from build123d import *


with BuildPart() as part:
    # Sketch1 → Revolve1 (revolve)
    with BuildSketch(Plane.XY):
        with BuildLine():
            Line((10.15, 9.35), (10.15, 11.15))
            ThreePointArc((10.15, 11.15), (9.608147545, 12.458147545), (8.3, 13))
            Line((8.3, 13), (8.3, 14))
            Line((8.3, 14), (0, 14))
            Line((0, 14), (0, 13))
            ThreePointArc((0, 13), (-1.308147545, 12.458147545), (-1.85, 11.15))
            Line((-1.85, 11.15), (-1.85, 9.35))
            ThreePointArc((-1.85, 9.35), (-1.308147545, 8.041852455), (0, 7.5))
            Line((0, 7.5), (0, 6.5))
            Line((0, 6.5), (8.3, 6.5))
            Line((8.3, 6.5), (8.3, 7.5))
            ThreePointArc((8.3, 7.5), (9.608147545, 8.041852455), (10.15, 9.35))
        make_face()
    revolve(axis=Axis((-8.833016473, 0, 0), (1, 0, 0)))


solid = part.part
Verification items for the finished model (mm, model axes). A direction names the side the tool comes from. Coordinates: 2 decimals unless noted, no trailing zeros. Order: outer loops, then holes, each group sorted by start corner. A loop starts at its lowest first (then second) coordinate and runs counter-clockwise, first axis right, second up. Notation, with made-up numbers: M 79.25,65.5 L 122.25,65.5 A24 cw 122.25,93.5 Z; hole C 2.5,26.25 d10. An arc over 180 degrees is marked long. One line per item, written item: value. Start each with the question number.
Item 1: Sectioned sample at C-C on x = 7.5. Record the cut outline in (y, z), then the cut area to 3 significant figures.
Item 2: Thickness scan on probe 1 along Z at (x, y) = (3.75, 0); probe 2 along X at (y, z) = (-3.5, -8.5); probe 3 along Y at (x, z) = (5.25, 3). Record the ranges inside material, lowest first.
Item 3: Access from +Z, -Z, +X, -X, +Y, -Y to the whole of each face (thin tool, end or side, straight path). Record for faces 1 (the cylindrical face through (4.208, -5.158, -3.955)), 2 (the flat face through (8.3, -9.3, -9.3)).
Item 4: Mould release check, pull along Z, two halves, no side actions. Record for faces 3 (the flat face through (0, -6, 3)), 4 (the cylindrical face through (4.092, 12.932, -5.362)), 5 (the flat face through (0, 9.3, -9.3)): pulls with the +Z half, pulls with the -Z half, needs draft (parallel to the pull), parting line crosses it, or undercut.
Item 5: Depth check by flat-ended pin: P1, Ø2, axis at x = 2, z = 8, coming from the +Y side; P2, Ø5, axis at x = 0.5, z = 0.5, coming from the -Y side; P3, Ø2, axis at x = 6, y = 4.5, coming from the +Z side; P4, Ø1, axis at x = 8, y = 11, coming from the -Z side. Enter the tip coordinate at first touch or a pass-through.
Item 6: Sectioned sample at A-A on y = 0. Record the cut outline in (x, z).
Calculated:
1. outline: C 0,0 d28; hole C 0,0 d13
1. area: 483 mm^2
2. probe 1: -14 to -6.5, 6.5 to 14
2. probe 2: -1.84 to 10.14
2. probe 3: -13.67 to -5.77, 5.77 to 13.67
3. face 1: +X, -X
3. face 2: +X
4. face 3: undercut
4. face 4: parting line crosses it
4. face 5: needs draft
5. P1: y = 12.12
5. P2: y = -14
5. P3: z = 13.56
5. P4: z = -9.26
6. outline: M -1.85,-11.15 A1.85 ccw 0,-13 L 0,-14 L 8.3,-14 L 8.3,-13 A1.85 ccw 10.15,-11.15 L 10.15,-9.35 A1.85 ccw 8.3,-7.5 L 8.3,-6.5 L 0,-6.5 L 0,-7.5 A1.85 ccw -1.85,-9.35 Z; M -1.85,9.35 A1.85 ccw 0,7.5 L 0,6.5 L 8.3,6.5 L 8.3,7.5 A1.85 ccw 10.15,9.35 L 10.15,11.15 A1.85 ccw 8.3,13 L 8.3,14 L 0,14 L 0,13 A1.85 ccw -1.85,11.15 Z
